from build123d import *

# Parameters (mm, degrees)
SKETCH018_R             = 12
PAD008_DEPTH            = 19
SKETCH019_W             = 14.3
SKETCH019_H             = 10
PAD009_DEPTH            = 16.3
SKETCH020_R             = 2.1
PAD010_DEPTH            = 1
PAD011_DEPTH            = 10
BODY004_PLACEMENT_ANGLE = 90


with BuildPart() as part:
    # Sketch018 → Pad008 (new body)
    with BuildSketch(Plane.XY):
        Circle(SKETCH018_R)
    extrude(amount=PAD008_DEPTH)

    # Sketch019 (on Face3 of Pad008) → Pad009 (join)
    with BuildSketch(Plane.XY.offset(19)):
        with Locations((0, -11.5)):
            Rectangle(SKETCH019_W, SKETCH019_H)
    extrude(amount=-PAD009_DEPTH)

    # Sketch020 (on Face3 of Pad009) → Pad010 (join)
    with BuildSketch(Plane.XY.offset(19)):
        with BuildLine():
            ThreePointArc((15.5, -3.5), (19, 0), (15.5, 3.5))
            Line((15.5, 3.5), (-15.5, 3.5))
            ThreePointArc((-15.5, 3.5), (-19, 0), (-15.5, -3.5))
            Line((-15.5, -3.5), (15.5, -3.5))
        make_face()
        with Locations((15.5, 0)):
            Circle(SKETCH020_R, mode=Mode.SUBTRACT)
        with Locations((-15.5, 0)):
            Circle(SKETCH020_R, mode=Mode.SUBTRACT)
    extrude(amount=-PAD010_DEPTH)

    # Sketch021 (on Face11 of Pad010) → Pad011 (join)
    with BuildSketch(Plane.XY.offset(19)):
        with BuildLine():
            ThreePointArc((-2, 8), (-2.5, 6.5), (-2, 5))
            Line((-2, 5), (2, 5))
            ThreePointArc((2, 5), (2.5, 6.5), (2, 8))
            Line((-2, 8), (2, 8))
        make_face()
    extrude(amount=PAD011_DEPTH)


with BuildPart() as part_1:
    # Body004 placement: moved
    add(part.part.moved(Location((57.5, 0, -4.5))).rotate(Axis((57.5, 0, -4.5), (0, 0, 1)), BODY004_PLACEMENT_ANGLE))


solid = part_1.part
Here's how the part is built. I have some questions about the finished solid (model axes, mm). A direction names the side the tool comes from. Coordinates: 2 decimals unless noted, no trailing zeros. Loops run counter-clockwise (first coordinate to the right, second up) from the corner with the lowest first, then second, coordinate; pieces in that order, holes last. Notation, with made-up numbers: (72, 48.25) -> (100, 48.25) arc R32 cw to (100, 81.25) -> close; hole circle Ø4 at (71.5, 43). An arc over 180 degrees is marked (long way). Use one line per item in the form item = value. Start each with the question number.
(1) If we section it at A-A (x = 57.5): Please give me the cut outline in (y, z), then the cut area to 3 significant figures.
(2) If we section it at D-D (x = 51.5): Please give me the cut outline in (y, z).
(3) On a 3-axis mill with a long thin cutter (end or side, diameter ignored), from which of +Z, -Z, +X, -X, +Y, -Y can I reach the whole of each face in a straight line? I mean faces 1 (the face through (49.5, 0, 19)), 2 (the face through (61, -14, 14)), 3 (the face through (52.5, 0, 19)), 4 (the face through (51, 2.5, 19.4)). Say none if no direction works.
(4) We'd pull the mould along X, two halves only. Please class faces 5 (the face through (71, 7.15, 6)), 6 (the face through (61, 13, 14)), 7 (the face through (59.55, -15.96, 14.01)), 8 (the face through (45.6, -1.56, 4.87)): pulls with the +X half, pulls with the -X half, needs draft (parallel to the pull), parting line crosses it, or undercut.
(5) If we section it at B-B (y = 0): Please give me the cut outline in (x, z).
(6) Will these pins go through, and if not, where does the flat tip stop? pin 1 (5 mm diameter, centred on x = 57.5, y = -15.5, fed in from -Z); pin 2 (3 mm diameter, centred on x = 70.5, z = 4, fed in from -Y); pin 3 (14 mm diameter, centred on x = 66, y = -1.5, fed in from +Z).
(7) Please list where these lines run through material, in increasing order: line 1 along Y through (x, z) = (57.5, 13.8); line 2 along X through (y, z) = (-15.5, 14.3); line 3 along Z through (x, y) = (59.75, -9.5).
(8) If we section it at C-C (y = 14.5): Please give me the cut outline in (x, z), then the cut area to 3 significant figures.
Verdict:
q1.outline = (-19, 13.5) -> (-17.6, 13.5) -> (-17.6, 14.5) -> (-19, 14.5) -> close; (-13.4, 13.5) -> (-12, 13.5) -> (-12, -4.5) -> (12, -4.5) -> (12, 13.5) -> (13.4, 13.5) -> (13.4, 14.5) -> (-13.4, 14.5) -> close; (17.6, 13.5) -> (19, 13.5) -> (19, 14.5) -> (17.6, 14.5) -> close
q1.area = 462 mm²
q2.outline = (-10.39, -4.5) -> (10.39, -4.5) -> (10.39, 14.5) -> (2.45, 14.5) -> (2.45, 24.5) -> (-2.45, 24.5) -> (-2.45, 14.5) -> (-10.39, 14.5) -> close
q3.face_1 = +Z, -X, +Y, -Y
q3.face_2 = +Z, -Z, +X, -Y
q3.face_3 = +Z, +X, +Y, -Y
q3.face_4 = +Z, +Y
q4.face_5 = needs draft
q4.face_6 = pulls with the +X half
q4.face_7 = undercut
q4.face_8 = parting line crosses it
q5.outline = (45.5, -4.5) -> (69.5, -4.5) -> (69.5, -1.8) -> (74, -1.8) -> (74, 14.5) -> (52.5, 14.5) -> (52.5, 24.5) -> (49.5, 24.5) -> (49.5, 14.5) -> (45.5, 14.5) -> close
q6.pin_1 = 13.5
q6.pin_2 = -7.15
q6.pin_3 = 14.5
q7.line_1 = -19 to -17.6, -13.4 to 13.4, 17.6 to 19
q7.line_2 = 54 to 55.4, 59.6 to 61
q7.line_3 = -4.5 to 14.5
q8.outline = (54, 13.5) -> (55.65, 13.5) -> (55.65, 14.5) -> (54, 14.5) -> close; (59.35, 13.5) -> (61, 13.5) -> (61, 14.5) -> (59.35, 14.5) -> close
q8.area = 3.31 mm²
